Autodesk Fusion 360 part; units mm, degrees
sketch "Sketch1" plane through (0, 0, 0) normal (0, 1, 0) x (1, 0, 0)
  line L0 (1, 0) -> (74, 0)
  line L1 (75, -1) -> (75, -55)
  line L2 (0, -55) -> (0, -1)
  circle A0 centre (4, -4) radius 2
  line L3 (2, -48) -> (2, -8)
  arc A1 (7.7004, -53.519) -> (2.481, -48.2996) centre (4, -52) ccw
  arc A2 (0, -51.9989) -> (0, -52.0011) centre (4, -52) ccw
  arc A3 (0, -55) -> (1, -56) centre (1, -55) ccw
  arc A4 (2.481, -48.2996) -> (2, -48) centre (2, -48.5359) ccw
  arc A5 (8, -54) -> (7.7004, -53.519) centre (7.4641, -54) ccw
  circle A6 centre (4, -52) radius 2
  circle A7 centre (71, -52) radius 2
  line L4 (67, -54) -> (8, -54)
  line L5 (73, -8) -> (73, -48)
  arc A8 (72.519, -48.2996) -> (67.2996, -53.519) centre (71, -52) ccw
  arc A9 (74, -56) -> (75, -55) centre (74, -55) ccw
  arc A10 (73, -48) -> (72.519, -48.2996) centre (73, -48.5359) ccw
  arc A11 (67.2996, -53.519) -> (67, -54) centre (67.5359, -54) ccw
  circle A12 centre (71, -4) radius 2
  arc A13 (75, -1) -> (74, 0) centre (74, -1) ccw
  arc A14 (67.2996, -2.481) -> (72.519, -7.7004) centre (71, -4) ccw
  arc A15 (67, -2) -> (67.2996, -2.481) centre (67.5359, -2) ccw
  arc A16 (72.519, -7.7004) -> (73, -8) centre (73, -7.4641) ccw
  arc A17 (2.481, -7.7004) -> (7.7004, -2.481) centre (4, -4) ccw
  arc A18 (2.481, -7.7004) -> (7.7004, -2.481) centre (4, -4) ccw
  arc A19 (1, 0) -> (0, -1) centre (1, -1) ccw
  arc A20 (2, -8) -> (2.481, -7.7004) centre (2, -7.4641) ccw
  arc A21 (7.7004, -2.481) -> (8, -2) centre (7.4641, -2) ccw
  line L6 (45.5, -2.4997) -> (45.5, -4)
  line L7 (29.5, -2.5) -> (29.5, -4)
  arc A22 (29.5, -2.5) -> (29, -2) centre (29, -2.5) ccw
  arc A23 (46, -2) -> (45.5, -2.5003) centre (46, -2.5) ccw
  line L8 (29, -2) -> (8, -2)
  line L9 (67, -2) -> (46, -2)
  arc A24 (29.5, -4) -> (33.5, -8) centre (33.5, -4) ccw
  arc A25 (41.5, -8) -> (45.5, -4) centre (41.5, -4) ccw
  arc A26 (41.5015, 0) -> (41.4985, 0) centre (41.5, -4) ccw
  line L10 (33.5, -8) -> (41.5, -8)
  circle A27 centre (33.5, -4) radius 2
  circle A28 centre (41.5, -4) radius 2
  line L11 (32.5, -56.5) -> (32.5, -65)
  line L12 (33.5, -66) -> (41.5, -66)
  line L13 (42.5, -65) -> (42.5, -56.5)
  line L14 (33.5, -66) -> (41.5, -66)
  line L15 (74, -56) -> (43, -56)
  line L16 (32, -56) -> (1, -56)
  arc A29 (32.5, -56.5) -> (32, -56) centre (32, -56.5) ccw
  arc A30 (43, -56) -> (42.5, -56.5) centre (43, -56.5) ccw
  arc A31 (32.5, -65) -> (33.5, -66) centre (33.5, -65) ccw
  arc A32 (41.5, -66) -> (42.5, -65) centre (41.5, -65) ccw
  line L17 (42.5, -65) -> (42.5, -64.0151)
  line L18 (32.5, -64.0151) -> (32.5, -65)
  line L19 (35, -64) -> (40, -64)
  line L20 (40, -63) -> (35, -63)
  line L21 (34.5, -62) -> (40.5, -62)
  line L22 (41.5, -63) -> (41.5, -64)
  line L23 (40.5, -65) -> (34.5, -65)
  line L24 (33.5, -64) -> (33.5, -63)
  arc A33 (34.5, -62) -> (33.5, -63) centre (34.5, -63) ccw
  arc A34 (40.5, -65) -> (41.5, -64) centre (40.5, -64) ccw
  arc A35 (40, -64) -> (40, -63) centre (40, -63.5) ccw
  arc A36 (41.5, -63) -> (40.5, -62) centre (40.5, -63) ccw
  arc A37 (33.5, -64) -> (34.5, -65) centre (34.5, -64) ccw
  arc A38 (35, -63) -> (35, -64) centre (35, -63.5) ccw
  dimension "d2" = 4
  dimension "d3" = 4
extrude "Extrude1" add sketch "Sketch1" along normal blind 1 makes body 1 at (36.5, 0, 58.3333) makes body 2 at (38.3333, 0, 63.6667)
extrude "Extrude2" add sketch "Sketch1" along normal blind 5 contours L21 L22 L23 L24 A33 A34 A36 A37 bodies 1 2
Read the model definition and answer for the solid it produces. Units are mm, in the model's axes. A direction names the side the tool comes from. Round coordinates to 2 decimals unless told otherwise and drop trailing zeros. Write each loop counter-clockwise with the first axis right and the second up, starting at its lowest first coordinate (ties: lowest second). Pieces come first, ordered by that corner, then holes.
1. Straight lines are drawn through the part: L1, parallel to Z at x = 4, y = 0.55; L2, parallel to Z at x = 33.5, y = 0.3; L3, parallel to X at y = 0.6, z = 37. For each, find the intervals that lie inside material, in ascending order.
2. Determine the mould class of faces 1 (the face through (71.923, 0.493, 50.226)), 2 (the face through (37, 3, 62)) for opening direction X: pulls with the +X half, pulls with the -X half, needs draft (parallel to the pull), parting line crosses it, or undercut.
3. The part is cut by section C-C, the plane y = 1.8. Determine the outline of the cut face in (x, z), then the cut area to 3 significant figures.
4. Which of the six approach directions +Z, -Z, +X, -X, +Y, -Y give full straight-line access (tool end or side, diameter ignored) to faces 3 (the face through (30.703, 0.493, 6.859)), 4 (the face through (38, 3, 63)), 5 (the face through (37, 0, 55)), 6 (the face through (38, 3, 65))?
5. The part is cut by section D-D, the plane z = 5. Determine the outline of the cut face in (x, y), then the cut area to 3 significant figures.
6. Given pin 1 Ø2 at (x, y) = (36, 2.5) entering from -Z; pin 2 Ø8 at (x, z) = (34, 13) entering from -Y; pin 3 Ø4.5 at (x, z) = (4, 4) entering from +Y; pin 4 Ø0.8 at (x, y) = (21.5, 0.5) entering from +Z, each flat-ended and moving along its own axis, determine where each tip first touches the part or whether it passes through.
7. The part is cut by section A-A, the plane x = 25. Determine the outline of the cut face in (y, z), then the cut area to 3 significant figures.
8. The part is cut by section B-B, the plane z = 47. Determine the outline of the cut face in (x, y), then the cut area to 3 significant figures.
Values:
1. L1: z = 0 to 2, 6 to 8, 48 to 50, 54 to 56
1. L2: z = 0 to 2, 6 to 8, 54 to 66
1. L3: x = 0 to 2, 73 to 75
2. face 1: undercut
2. face 2: needs draft
3. outline: (33.5, 63) arc R1 ccw to (34.5, 62) - (40.5, 62) arc R1 ccw to (41.5, 63) - (41.5, 64) arc R1 ccw to (40.5, 65) - (34.5, 65) arc R1 ccw to (33.5, 64) - close; hole (35, 63) - (40, 63) arc R0.5 ccw to (40, 64) - (35, 64) arc R0.5 ccw to start
3. area: 17.4 mm2
4. face 3: +Y, -Y
4. face 4: +Y
4. face 5: +Z, -Z, +X, -X, -Y
4. face 6: +Z, +X, -X, +Y
5. outline: (0, 0) - (2.27, 0) - (2.27, 1) - (0, 1) - close; (5.73, 0) - (7.87, 0) - (7.87, 1) - (5.73, 1) - close; (29.63, 0) - (31.77, 0) - (31.77, 1) - (29.63, 1) - close; (35.23, 0) - (39.77, 0) - (39.77, 1) - (35.23, 1) - close; (43.23, 0) - (45.37, 0) - (45.37, 1) - (43.23, 1) - close; (67.13, 0) - (69.27, 0) - (69.27, 1) - (67.13, 1) - close; (72.73, 0) - (75, 0) - (75, 1) - (72.73, 1) - close
5. area: 17.6 mm2
6. pin 1: stops at z = 62
6. pin 2: passes through
6. pin 3: stops at y = 1
6. pin 4: stops at z = 56
7. outline: (0, 0) - (1, 0) - (1, 2) - (0, 2) - close; (0, 54) - (1, 54) - (1, 56) - (0, 56) - close
7. area: 4.00 mm2
8. outline: (0, 0) - (2, 0) - (2, 1) - (0, 1) - close; (73, 0) - (75, 0) - (75, 1) - (73, 1) - close
8. area: 4.00 mm2
